Check sheet for the modelled part. Datum: model origin and axes. Units: mm. A direction names the side the tool comes from. Round coordinates to 2 decimals unless told otherwise and drop trailing zeros. Loops run counter-clockwise (first coordinate to the right, second up) from the corner with the lowest first, then second, coordinate; pieces in that order, holes last. Notation, with made-up numbers: (-37, 18) -> (7, 18) arc R31 ccw to (7, 57) -> close; hole circle Ø6 at (-4, 66). An arc over 180 degrees is marked (long way). Return JSON: item names as keys, results as strings.
Autodesk Inventor part; units mm, degrees
ref_plane "YZ Plane" through (0, 0, 0) normal (1, 0, 0) x (0, 1, 0)
ref_plane "XZ Plane" through (0, 0, 0) normal (0, 1, 0) x (-1, 0, 0)
ref_plane "XY Plane" through (0, 0, 0) normal (0, 0, 1) x (1, 0, 0)
sketch "Boceto1" plane through (0, 0, 0) normal (0, 1, 0) x (-1, 0, 0)
  circle A0 centre (0, 0) radius 7.5 construction
  line L0 (0, 7.5) -> (4.5449, 13.2126)
  arc A1 (9.17, 10.5423) -> (4.5449, 13.2126) centre (6.6578, 11.5316) ccw
  line L1 (9.17, 10.5423) -> (6.4952, 3.75)
  line L2 (6.4952, 3.75) -> (13.7149, 2.6703)
  arc A2 (13.7149, -2.6703) -> (13.7149, 2.6703) centre (13.3156, 0) ccw
  line L3 (13.7149, -2.6703) -> (6.4952, -3.75)
  line L4 (6.4952, -3.75) -> (9.17, -10.5423)
  arc A3 (4.5449, -13.2126) -> (9.17, -10.5423) centre (6.6578, -11.5316) ccw
  line L5 (4.5449, -13.2126) -> (0, -7.5)
  line L6 (0, -7.5) -> (-4.5449, -13.2126)
  arc A4 (-9.17, -10.5423) -> (-4.5449, -13.2126) centre (-6.6578, -11.5316) ccw
  line L7 (-9.17, -10.5423) -> (-6.4952, -3.75)
  line L8 (-6.4952, -3.75) -> (-13.7149, -2.6703)
  arc A5 (-13.7149, 2.6703) -> (-13.7149, -2.6703) centre (-13.3156, 0) ccw
  line L9 (-13.7149, 2.6703) -> (-6.4952, 3.75)
  line L10 (-6.4952, 3.75) -> (-9.17, 10.5423)
  line L11 (0, 7.5) -> (-4.5449, 13.2126)
  arc A6 (-4.5449, 13.2126) -> (-9.17, 10.5423) centre (-6.6578, 11.5316) ccw
  dimension "d6" = 15
  dimension "d11" = 2.7
  dimension "d12" = 7.3
  dimension "d13" = 60
sketch "Boceto2" plane through (0, 0, 0) normal (0, 1, 0) x (-1, 0, 0)
  line L0 (17.6656, 17.6656) -> (-17.6656, 17.6656)
  line L1 (-17.6656, 17.6656) -> (-17.6656, -17.6656)
  line L2 (-17.6656, -17.6656) -> (17.6656, -17.6656)
  line L3 (17.6656, -17.6656) -> (17.6656, 17.6656)
  arc A0 (-13.7149, 2.6703) -> (-13.7149, -2.6703) centre (-13.3156, 0) ccw
  point P0 (0, 0)
  point P1 (0, -17.6656)
  point P2 (17.6656, 0)
  dimension "d14" = 4.35
  dimension "profundidad_hombro" = 35.3311
extrude "Extrusión1" add sketch "Boceto2" against normal blind 7.55
extrude "Extrusión2" cut sketch "Boceto1" against normal blind 4
sketch "Boceto3" plane through (0, -7.55, 0) normal (0, -1, 0) x (1, 0, 0)
  line L0 (17.6656, -17.6656) -> (-17.6656, -17.6656) construction
  line L1 (-8.8344, 17.6656) -> (17.6656, 17.6656)
  line L2 (17.6656, 17.6656) -> (17.6656, 1.6656)
  line L3 (17.6656, 1.6656) -> (-8.8344, 1.6656)
  line L4 (-8.8344, 1.6656) -> (-8.8344, 17.6656)
  line L5 (17.6656, 17.6656) -> (-17.6656, 17.6656)
  line L6 (17.6656, 17.6656) -> (-17.6656, 17.6656)
  line L7 (-17.6656, 17.6656) -> (-17.6656, -17.6656)
  line L8 (-17.6656, -17.6656) -> (17.6656, -17.6656)
  line L9 (17.6656, -17.6656) -> (17.6656, 17.6656)
  point P0 (0, 0)
  point P1 (-2.7738, 1.6656)
  dimension "d20" = 16
  dimension "d59" = 26.5
extrude "Extrusión3" add sketch "Boceto3" along normal blind 48.5 contours L1 L2 L3 L4
sketch "Boceto4" plane through (0, -56.05, 0) normal (0, -1, 0) x (1, 0, 0)
  line L0 (17.6656, 17.6656) -> (17.6656, -17.6656)
  line L1 (-17.6656, -17.6656) -> (17.6656, -17.6656)
  line L2 (17.6656, -17.6656) -> (17.6656, 17.6656)
  line L3 (17.6656, 17.6656) -> (-17.6656, 17.6656)
  line L4 (-17.6656, 17.6656) -> (-17.6656, -17.6656)
  point P0 (0, 0)
extrude "Extrusión4" add sketch "Boceto4" along normal blind 5
sketch "Boceto5" plane through (0, -61.05, 0) normal (0, -1, 0) x (1, 0, 0)
  circle A0 centre (0, 0) radius 10
  dimension "diametro_eje_hombro" = 20
extrude "Extrusión5" add sketch "Boceto5" along normal blind 18
sketch "Sketch11" plane through (-17.6656, 0, 17.6656) normal (0, 0, 1) x (1, 0, 0)
  line L0 (11.8311, -52.05) -> (32.3311, -52.05)
  line L1 (32.3311, -52.05) -> (32.3311, -11.55)
  line L2 (32.3311, -11.55) -> (11.8311, -11.55)
  line L3 (11.8311, -11.55) -> (11.8311, -52.05)
  line L4 (8.8311, -7.55) -> (8.8311, -56.05)
  line L5 (35.3311, 0) -> (35.3311, -61.05)
  point P0 (17.6656, 0)
  point P1 (11.8311, -31.8)
  point P2 (8.8311, -31.8)
  dimension "d60" = 40.5
  dimension "d61" = 3
  dimension "d62" = 3
extrude "Extrusion12" cut sketch "Sketch11" against normal up to surface (16 mm away)
sketch "Sketch12" plane through (-17.6656, 0, 17.6656) normal (0, 0, 1) x (1, 0, 0)
  circle A0 centre (16.8311, -56) radius 1.55
  circle A1 centre (27.3311, -56) radius 1.55
  circle A2 centre (27.3311, -7.6) radius 1.55
  circle A3 centre (16.8311, -7.6) radius 1.55
  line L0 (32.3311, -52.05) -> (11.8311, -52.05)
  line L1 (11.8311, -11.55) -> (32.3311, -11.55)
  line L2 (32.3311, -11.55) -> (32.3311, -52.05)
  line L3 (11.8311, -52.05) -> (11.8311, -11.55)
  point P0 (17.6656, 0)
  dimension "d65" = 3.1
  dimension "d66" = 3.95
  dimension "d67" = 3.95
  dimension "d68" = 5
  dimension "d69" = 5
extrude "Extrusion13" cut sketch "Sketch12" against normal blind 14 contours A0 | A1 | A2 | A3
fillet "Fillet2" radius 12 2 edges at (17.6656, -3.775, -17.6656) (17.6656, -58.55, -17.6656)
fillet "Fillet3" radius 3 5 edges at (-10, -61.05, 0) (-17.6656, -58.55, 17.6656) (-17.6656, -3.775, 17.6656) (-17.6656, -3.775, -17.6656) (-17.6656, -58.55, -17.6656)
sketch "Sketch15" plane through (0, -4, 0) normal (0, 1, 0) x (1, 0, 0)
  arc A0 (-4.5449, 13.2126) -> (-9.17, 10.5423) centre (-6.6578, 11.5316) ccw
  circle A1 centre (-6.6578, 11.5316) radius 1.2
  arc A2 (9.17, 10.5423) -> (4.5449, 13.2126) centre (6.6578, 11.5316) ccw
  circle A3 centre (6.6578, 11.5316) radius 1.2
  point P0 (0, 0)
  dimension "d78" = 1.5
extrude "Extrusion15" cut sketch "Sketch15" against normal blind 10
equation "\"d12\" = largo_petalo"
equation "\"d62\" = d61"
equation "\"d67\" = d66"
properties part number "Pata - Hombro"
Q1. Section check D-D (y = -59). Record the boundary of the cut face in (x, z).
Results list:
{"outline": "(-17.67, -14.67) arc R3 ccw to (-14.67, -17.67) -> (5.67, -17.67) arc R12 ccw to (17.67, -5.67) -> (17.67, 17.67) -> (-14.67, 17.67) arc R3 ccw to (-17.67, 14.67) -> close"}
Q2. Section check C-C (z = 15.5). Record the boundary of the cut face in (x, y).
Results list:
{"outline": "(-17.55, -61.05) -> (17.67, -61.05) -> (17.67, 0) -> (-17.55, 0) -> (-17.55, -7.55) -> (-8.83, -7.55) -> (-8.83, -56.05) -> (-17.55, -56.05) -> close; hole (-5.83, -52.05) -> (14.67, -52.05) -> (14.67, -11.55) -> (-5.83, -11.55) -> close; hole circle Ø3.1 at (-0.83, -56); hole circle Ø3.1 at (-0.83, -7.6); hole circle Ø3.1 at (9.67, -56); hole circle Ø3.1 at (9.67, -7.6)"}
Q3. Section check A-A (y = -37.5). Record the boundary of the cut face in (x, z), then the cut area to 3 significant figures.
Results list:
{"outline": "(-8.83, 1.67) -> (-5.83, 1.67) -> (-5.83, 17.67) -> (-8.83, 17.67) -> close; (14.67, 1.67) -> (17.67, 1.67) -> (17.67, 17.67) -> (14.67, 17.67) -> close", "area": "96.0 mm^2"}
Q4. Section check B-B (z = 0). Record the boundary of the cut face in (x, y).
Results list:
{"outline": "(-17.67, -61.05) -> (-13, -61.05) arc R3 cw to (-10, -64.05) -> (-10, -79.05) -> (10, -79.05) -> (10, -64.05) arc R3 cw to (13, -61.05) -> (17.67, -61.05) -> (17.67, -56.05) -> (-17.67, -56.05) -> close; (-17.67, -7.55) -> (17.67, -7.55) -> (17.67, 0) -> (16.02, 0) -> (16.02, -4) -> (-16.02, -4) -> (-16.02, 0) -> (-17.67, 0) -> close"}
Q5. Draft check along Y on faces 1 (the flat face through (-1, -56, 3.666)), 2 (the flat face through (0, -79.05, 0)), 3 (the cylindrical face through (-16.015, -1.972, -0.054)). Enter one of: released by +Y, released by -Y, zero draft, split by the parting line, or undercut.
Results list:
{"face 1": "undercut", "face 2": "released by -Y", "face 3": "zero draft"}
Q6. Tool access check on faces 4 (the flat face through (4, -52.05, 10)), 5 (the flat face through (10, -56, 3.666)), 6 (the cylindrical face through (-6.92, -5.75, -10.36)), 7 (the flat face through (-17.666, -59, 0)). Record the directions out of +Z, -Z, +X, -X, +Y, -Y that give a thin tool (end or side, any length) a straight path to the whole face; none if there is none.
Results list:
{"face 4": "+Z, -Z", "face 5": "+Z", "face 6": "+Y", "face 7": "+Z, -Z, -X, +Y, -Y"}
Q7. Material ranges on line 1 (X direction, y = -37, z = 16.5); line 2 (Y direction, x = 4, z = 4); line 3 (Y direction, x = -8.5, z = 1), recorded low to high.
Results list:
{"line 1": "-8.83 to -5.83, 14.67 to 17.67", "line 2": "-79.05 to -52.05, -11.55 to -4", "line 3": "-79.05 to -56.05, -7.55 to -4"}
Q8. Go/stop test with flat-tipped pins: pin 1 (5 mm diameter, centred on x = 9.67, y = -7.6, fed in from +Z); pin 2 (1.9 mm diameter, centred on x = 6.66, z = -11.53, fed in from +Y); pin 3 (1.5 mm diameter, centred on y = -53.5, z = 5, fed in from -X); pin 4 (0.9 mm diameter, centred on x = -1, y = -7.5, fed in from +Z). Record where each tip stops, or that it passes through.
Results list:
{"pin 1": "z = 17.67", "pin 2": "y = -56.05", "pin 3": "x = -8.83", "pin 4": "z = 3.67"}
